from build123d import *

# Parameters (mm, degrees)
SKETCH1_R           = 1.5
SKETCH1_R_2         = 0.586127488
SKETCH1_R_3         = 0.42585763
BOSS_EXTRUDE1_DEPTH = 2
SKETCH3_R           = 0.579621875
CUT_EXTRUDE1_DEPTH  = 2
SKETCH4_R           = 0.5
BOSS_EXTRUDE3_DEPTH = 2


with BuildPart() as part:
    # Sketch1 → Boss-Extrude1 (new body)
    with BuildSketch(Plane(origin=(0, 0, 0), x_dir=(1, 0, 0), z_dir=(0, 1, 0))):
        with BuildLine():
            Line((-5.704810184, -3.532312602), (0.0197897, -3.499944052))
            ThreePointArc((0.0197897, -3.499944052), (1.899950502, -2.939419686), (3.183109291, -1.455271536))
            Line((3.183109291, -1.455271536), (6.127465187, 4.984905694))
            ThreePointArc((6.127465187, 4.984905694), (4.399627432, 9.62328652), (-0.238753394, 7.895448766))
            Line((-0.238753394, 7.895448766), (-1.72322244, 4.648475885))
            ThreePointArc((-1.72322244, 4.648475885), (-2.456456033, 3.800391228), (-3.530833635, 3.48009159))
            Line((-3.530833635, 3.48009159), (-5.744389584, 3.467575502))
            ThreePointArc((-5.744389584, 3.467575502), (-9.224543936, -0.05215825), (-5.704810184, -3.532312602))
        make_face()
        with Locations(Location((0, 0, 0), (0, 0, 270))):
            Circle(SKETCH1_R, mode=Mode.SUBTRACT)
        with Locations(Location((-5.724599884, -0.03236855, 0), (0, 0, 270))):
            Circle(SKETCH1_R_2, mode=Mode.SUBTRACT)
        with Locations(Location((2.944355896, 6.44017723, 0), (0, 0, 270))):
            Circle(SKETCH1_R_3, mode=Mode.SUBTRACT)
    extrude(amount=BOSS_EXTRUDE1_DEPTH)

    # Sketch3 → Cut-Extrude1 (cut)
    with BuildSketch(Plane(origin=(0, 2, 0), x_dir=(1, 0, 0), z_dir=(0, 1, 0))):
        with Locations(Location((2.073730064, 4.551378241, 0), (0, 0, 270))):
            Circle(SKETCH3_R)
    extrude(amount=-CUT_EXTRUDE1_DEPTH, mode=Mode.SUBTRACT)

    # Sketch4 → Boss-Extrude3 (add)
    with BuildSketch(Plane(origin=(0, 2, 0), x_dir=(1, 0, 0), z_dir=(0, 1, 0))):
        with BuildLine():
            Line((13.583389447, 11.376075771), (6.127465187, 4.984905694))
            Line((6.127465187, 4.984905694), (0.873997954, 9.262165534))
            Line((0.873997954, 9.262165534), (7.997134718, 13.945290547))
            ThreePointArc((7.997134718, 13.945290547), (12.795032794, 17.01966473), (13.583389447, 11.376075771))
        make_face()
        with Locations(Location((11.381075149, 13.945290547, 0), (0, 0, 270))):
            Circle(SKETCH4_R, mode=Mode.SUBTRACT)
    extrude(amount=-BOSS_EXTRUDE3_DEPTH)


solid = part.part
Geometry check sheet. Reference: the model listing, model coordinates, mm. Give positions to 0.01 mm unless a question says otherwise; leave off trailing zeros. Order: outer loops, then holes, each group sorted by start corner. A loop starts at its lowest first (then second) coordinate and runs counter-clockwise, first axis right, second up.
1) Cross-section at C-C (z = -8.75). Record the boundary of the cut face in (x, y).
Results are:
outline: (0.31, 0) - (10.52, 0) - (10.52, 2) - (0.31, 2) - close
2) Material ranges on probe 1 along X at (y, z) = (0.75, 0); probe 2 along X at (y, z) = (1.45, -14); probe 3 along Z at (x, y) = (11.5, 1.75), recorded low to high.
Results are:
probe 1: x = -9.22 to -6.31, -5.14 to -1.5, 1.5 to 3.85
probe 2: x = 8 to 10.88, 11.88 to 14.76
probe 3: z = -17.33 to -14.43, -13.46 to -9.59
3) Gauge pin test, flat ends, axial feed: pin 1 (0.9 mm diameter, centred on x = 2.07, z = -4.55, fed in from -Y); pin 2 (6 mm diameter, centred on x = 11.5, z = -9.5, fed in from +Y). Record the tip position at first contact, or that the pin passes through.
Results are:
pin 1: passes through
pin 2: stops at y = 2
4) Draft check along Z on faces 1 (the cylindrical face through (1.51, 1.01, -4.68)), 2 (the cylindrical face through (-2.44, 0.99, -3.81)), 3 (the flat face through (2.94, 2, -7.04)). Enter one of: released by +Z, released by -Z, zero draft, split by the parting line, or undercut.
Results are:
face 1: undercut
face 2: released by -Z
face 3: zero draft
5) Cross-section at D-D (x = 10.25). Record the boundary of the cut face in (y, z), then the cut area to 3 significant figures.
Results are:
outline: (0, -17.13) - (2, -17.13) - (2, -8.52) - (0, -8.52) - close
area: 17.2 mm2
6) Cross-section at B-B (y = 0.65). Record the boundary of the cut face in (x, z), then the cut area to 3 significant figures.
Results are:
outline: (-5.74, -3.47) - (-3.53, -3.48) arc R2 cw to (-1.72, -4.65) - (-0.24, -7.9) arc R3.5 ccw to (1.17, -9.46) - (8, -13.95) arc R3.38 ccw (long way) to (13.58, -11.38) - (6.13, -4.98) - (3.18, 1.46) arc R3.5 ccw to (0.02, 3.5) - (-5.7, 3.53) arc R3.5 ccw to start; hole circle Ø1.17 at (-5.72, 0.03); hole circle Ø3 at (0, 0); hole circle Ø1.16 at (2.07, -4.55); hole circle Ø0.85 at (2.94, -6.44); hole circle Ø1 at (11.38, -13.95)
area: 186 mm2
7) Cross-section at A-A (z = 0). Record the boundary of the cut face in (x, y).
Results are:
outline: (-9.22, 0) - (-6.31, 0) - (-6.31, 2) - (-9.22, 2) - close; (-5.14, 0) - (-1.5, 0) - (-1.5, 2) - (-5.14, 2) - close; (1.5, 0) - (3.85, 0) - (3.85, 2) - (1.5, 2) - close
